Model file for the job. Use its own axes, mm. A direction names the side the tool comes from. Round coordinates to 2 decimals unless told otherwise and drop trailing zeros. Order: outer loops, then holes, each group sorted by start corner. A loop starts at its lowest first (then second) coordinate and runs counter-clockwise, first axis right, second up. Notation, with made-up numbers: M -23,55 L 31,55 A19 cw 31,61 Z; hole C -38,72.5 d6. An arc over 180 degrees is marked long. Return JSON: item names as keys, results as strings. Group by question number.
Item 1: Pull direction Y, two halves, no side cores. Call faces 3 (the face through (28, 56, -10)), 4 (the face through (107, 30, -5)), 5 (the face through (28, -8, -20.01)): pulls with the +Y half, pulls with the -Y half, needs draft (parallel to the pull), parting line crosses it, or undercut.
Item 2: Slice it at C-C on z = -4.25. Give the number of separate pieces and of enclosed holes in the cut face, then the cut area to 3 significant figures.
Item 3: Probe line 1 along Y through (x, z) = (-36, -7.5); line 2 along X through (y, z) = (-29.5, -3); line 3 along Y through (x, z) = (76, -8). List the from-to ranges inside material, lowest first.
Item 4: Pin check, flat tip, straight feed: pin 1 Ø1 at (x, y) = (-47, 35) entering from +Z. Stop position of the tip, or through.
Item 5: Slice it at A-A on x = -4. Write the cut outline in (y, z).
Item 6: Which spindle directions (+Z, -Z, +X, -X, +Y, -Y) get a long thin tool onto all of the face, cutting with end or side? Do faces 1 (the face through (-100, -10, -10)), 2 (the face through (81, 25, -5)). Say none if no direction does.
Item 7: Slice it at B-B on y = -19. Write the cut outline in (x, z).
from build123d import *

# Parameters (mm, degrees)
BOX013_W               = 120
BOX013_H               = 66
BOX013_DEPTH           = 10
BOX002_W               = 14
BOX002_H               = 18
BOX002_DEPTH           = 10
BOX003_W               = 14
BOX003_H               = 18
BOX003_DEPTH           = 10
BOX004_W               = 14
BOX004_H               = 18
BOX004_DEPTH           = 10
BOX005_W               = 14
BOX005_H               = 18
BOX005_DEPTH           = 10
BOX006_W               = 33
BOX006_H               = 2
BOX006_DEPTH           = 10
BOX006_PLACEMENT_ANGLE = 90
BOX009_W               = 33
BOX009_H               = 2
BOX009_DEPTH           = 10
BOX009_PLACEMENT_ANGLE = 90
BOX010_W               = 33
BOX010_H               = 2
BOX010_DEPTH           = 10
BOX010_PLACEMENT_ANGLE = 90
BOX015_W               = 14
BOX015_H               = 18
BOX015_DEPTH           = 10
BOX022_W               = 14
BOX022_H               = 18
BOX022_DEPTH           = 10
BOX001_W               = 124
BOX001_H               = 2
BOX001_DEPTH           = 10
BOX_W                  = 260
BOX_H                  = 130
BOX_DEPTH              = 20
FILLET004_R            = 1
FILLET_R               = 1


with BuildPart() as cube003:
    # Box013 → Box013 (new body)
    with BuildSketch(Plane(origin=(-60, -48, -9), x_dir=(1, 0, 0), z_dir=(0, 0, 1))):
        with Locations((60, 33)):
            Rectangle(BOX013_W, BOX013_H)
    extrude(amount=BOX013_DEPTH)


with BuildPart() as obj1:
    # Box002 → Box002 (new body)
    with BuildSketch(Plane(origin=(8, 25, -9), x_dir=(1, 0, 0), z_dir=(0, 0, 1))):
        with Locations((7, 9)):
            Rectangle(BOX002_W, BOX002_H)
    extrude(amount=BOX002_DEPTH)


with BuildPart() as obj2:
    # Box003 → Box003 (new body)
    with BuildSketch(Plane(origin=(-22, 25, -9), x_dir=(1, 0, 0), z_dir=(0, 0, 1))):
        with Locations((7, 9)):
            Rectangle(BOX003_W, BOX003_H)
    extrude(amount=BOX003_DEPTH)


with BuildPart() as obj3:
    # Box004 → Box004 (new body)
    with BuildSketch(Plane(origin=(-52, 25, -9), x_dir=(1, 0, 0), z_dir=(0, 0, 1))):
        with Locations((7, 9)):
            Rectangle(BOX004_W, BOX004_H)
    extrude(amount=BOX004_DEPTH)


with BuildPart() as obj4:
    # Box005 → Box005 (new body)
    with BuildSketch(Plane(origin=(-82, 25, -9), x_dir=(1, 0, 0), z_dir=(0, 0, 1))):
        with Locations((7, 9)):
            Rectangle(BOX005_W, BOX005_H)
    extrude(amount=BOX005_DEPTH)


with BuildPart() as obj5:
    # Box006 → Box006 (new body)
    with BuildSketch(Plane.XY):
        with Locations((16.5, 1)):
            Rectangle(BOX006_W, BOX006_H)
    extrude(amount=BOX006_DEPTH)


with BuildPart() as obj5_1:
    # Box006 placement: moved
    add(obj5.part.moved(Location((107, 14, -9))).rotate(Axis((107, 14, -9), (0, 0, 1)), BOX006_PLACEMENT_ANGLE))


with BuildPart() as obj6:
    # Box009 → Box009 (new body)
    with BuildSketch(Plane.XY):
        with Locations((16.5, 1)):
            Rectangle(BOX009_W, BOX009_H)
    extrude(amount=BOX009_DEPTH)


with BuildPart() as obj6_1:
    # Box009 placement: moved
    add(obj6.part.moved(Location((128, 14, -9))).rotate(Axis((128, 14, -9), (0, 0, 1)), BOX009_PLACEMENT_ANGLE))


with BuildPart() as obj7:
    # Box010 → Box010 (new body)
    with BuildSketch(Plane.XY):
        with Locations((16.5, 1)):
            Rectangle(BOX010_W, BOX010_H)
    extrude(amount=BOX010_DEPTH)


with BuildPart() as obj7_1:
    # Box010 placement: moved
    add(obj7.part.moved(Location((149, 14, -9))).rotate(Axis((149, 14, -9), (0, 0, 1)), BOX010_PLACEMENT_ANGLE))


with BuildPart() as obj8:
    # Box015 → Box015 (new body)
    with BuildSketch(Plane(origin=(74, 25, -9), x_dir=(1, 0, 0), z_dir=(0, 0, 1))):
        with Locations((7, 9)):
            Rectangle(BOX015_W, BOX015_H)
    extrude(amount=BOX015_DEPTH)


with BuildPart() as obj9:
    # Box022 → Box022 (new body)
    with BuildSketch(Plane(origin=(37, 25, -9), x_dir=(1, 0, 0), z_dir=(0, 0, 1))):
        with Locations((7, 9)):
            Rectangle(BOX022_W, BOX022_H)
    extrude(amount=BOX022_DEPTH)


with BuildPart() as holes:
    # Box001 → Box001 (new body)
    with BuildSketch(Plane(origin=(-62, -61, -8), x_dir=(1, 0, 0), z_dir=(0, 0, 1))):
        with Locations((62, 1)):
            Rectangle(BOX001_W, BOX001_H)
    extrude(amount=BOX001_DEPTH)

    # Fusion: union obj1, obj2, obj3, obj4, obj5, obj6, obj7, obj8, obj9
    add(obj1.part)
    add(obj2.part)
    add(obj3.part)
    add(obj4.part)
    add(obj5_1.part)
    add(obj6_1.part)
    add(obj7_1.part)
    add(obj8.part)
    add(obj9.part)


with BuildPart() as box:
    # Box → Box (new body)
    with BuildSketch(Plane(origin=(-100, -74, -20.01), x_dir=(1, 0, 0), z_dir=(0, 0, 1))):
        with Locations((130, 65)):
            Rectangle(BOX_W, BOX_H)
    extrude(amount=BOX_DEPTH)

    # Fillet004
    fillet004_edges = [box.edges().sort_by_distance(p)[0] for p in [
        (-100, -74, -10.01),
        (-100, -9, -0.01),
        (-100, 56, -10.01),
        (-100, -9, -20.01),
        (160, -74, -10.01),
        (160, -9, -0.01),
        (160, 56, -10.01),
        (160, -9, -20.01),
        (30, -74, -20.01),
        (30, -74, -0.01),
        (30, 56, -20.01),
        (30, 56, -0.01),
    ]]
    fillet(fillet004_edges, radius=FILLET004_R)

    # Cut016: cut Holes
    add(holes.part, mode=Mode.SUBTRACT)

    # Cut: cut Cube003
    add(cube003.part, mode=Mode.SUBTRACT)

    # Fillet
    fillet_edges = [box.edges().sort_by_distance(p)[0] for p in [
        (0, -48, -0.01),
        (60, -15, -0.01),
        (0, 18, -0.01),
        (-60, -15, -0.01),
    ]]
    fillet(fillet_edges, radius=FILLET_R)


solid = box.part
Output values:
{
 "1": {"face 3": "pulls with the +Y half", "face 4": "undercut", "face 5": "needs draft"},
 "2": {"separate pieces": "1", "enclosed holes": "11", "area": "23,900 mm²"},
 "3": {"line 1": "-74 to -61, -59 to -48, 18 to 56", "line 2": "-100 to -60, 60 to 160", "line 3": "-74 to 25, 43 to 56"},
 "4": {"pin 1": "z = -9"},
 "5": {"outline": "M -74,-19.01 A1 ccw -73,-20.01 L 55,-20.01 A1 ccw 56,-19.01 L 56,-1.01 A1 ccw 55,-0.01 L 19,-0.01 A1 ccw 18,-1.01 L 18,-9 L -48,-9 L -48,-1.01 A1 ccw -49,-0.01 L -59,-0.01 L -59,-8 L -61,-8 L -61,-0.01 L -73,-0.01 A1 ccw -74,-1.01 Z"},
 "6": {"face 1": "+Z, -Z, -X, +Y, -Y", "face 2": "+Z"},
 "7": {"outline": "M -100,-19.01 A1 ccw -99,-20.01 L 159,-20.01 A1 ccw 160,-19.01 L 160,-1.01 A1 ccw 159,-0.01 L 61,-0.01 A1 ccw 60,-1.01 L 60,-9 L -60,-9 L -60,-1.01 A1 ccw -61,-0.01 L -99,-0.01 A1 ccw -100,-1.01 Z"}
}
